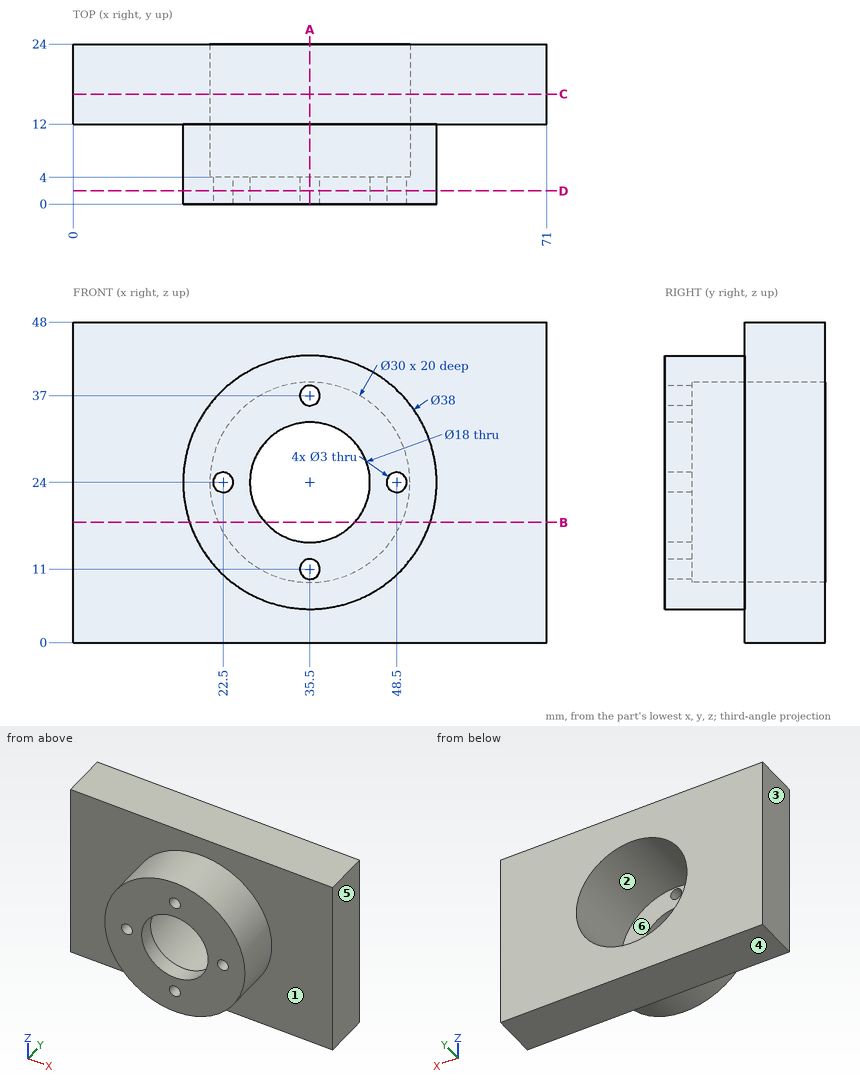
Input: dimensioned drawing with shaded views. Units: mm. Origin: part minimum x, y, z. A direction names the side the tool comes from. Give positions to 0.01 mm unless a question says otherwise; leave off trailing zeros. Write each loop counter-clockwise with the first axis right and the second up, starting at its lowest first coordinate (ties: lowest second). Pieces come first, ordered by that corner, then holes. Notation, with made-up numbers: (-32, 79) -> (-2, 79) arc R6 cw to (-2, 90) -> close; hole circle Ø8 at (45, 19.5). An arc over 180 degrees is marked (long way). Return JSON: item names as keys, results as strings. Group by question number.
1. Section B-B, the plane z = 18. Output: boundary loops of the cut face in (x, y), then the cut area to 3 significant figures.
2. Material intervals for line 1 (Z direction, x = 35.5, y = 1.15); line 2 (Z direction, x = 35.5, y = 16); line 3 (Y direction, x = 11, z = 20), sorted ascending. Write a range as from..to.
3. Section D-D, the plane y = 2. Output: boundary loops of the cut face in (x, z).
4. Section C-C, the plane y = 16.5. Output: boundary loops of the cut face in (x, z).
5. Mould query, pull axis X, two halves, no side actions, for the marked faces 4, 5 and 6. Classes: +X half, -X half, draft (parallel to the pull), parting line (faces both ways), or undercut.
6. Access query for the marked faces 1, 2 and 3. Directions: +Z, -Z, +X, -X, +Y, -Y. A direction counts if a zero-diameter tool reaches every point of the face in a straight line with its end or side. Return the directions, or none.
7. Pin query (flat end, axial travel): pin 1 Ø3.5 at (x, z) = (35.5, 11) entering from +Y; pin 2 Ø3 at (x, y) = (31, 5.5) entering from +Z; pin 3 Ø5 at (x, y) = (39.5, 5) entering from +Z. Return the tip coordinate at first contact, or that it passes through.
8. Section A-A, the plane x = 35.5. Output: boundary loops of the cut face in (y, z), then the cut area to 3 significant figures.
Determined:
{
 "1": {"outline": "(0, 12) -> (17.47, 12) -> (17.47, 0) -> (28.79, 0) -> (28.79, 4) -> (21.75, 4) -> (21.75, 24) -> (0, 24) -> close; (42.21, 0) -> (53.53, 0) -> (53.53, 12) -> (71, 12) -> (71, 24) -> (49.25, 24) -> (49.25, 4) -> (42.21, 4) -> close", "area": "681 mm2"},
 "2": {"line 1": "z = 5..9.5, 12.5..15, 33..35.5, 38.5..43", "line 2": "z = 0..9, 39..48", "line 3": "y = 12..24"},
 "3": {"outline": "circle Ø38 at (35.5, 24); hole circle Ø3 at (22.5, 24); hole circle Ø18 at (35.5, 24); hole circle Ø3 at (35.5, 11); hole circle Ø3 at (35.5, 37); hole circle Ø3 at (48.5, 24)"},
 "4": {"outline": "(0, 0) -> (71, 0) -> (71, 48) -> (0, 48) -> close; hole circle Ø30 at (35.5, 24)"},
 "5": {"face 4": "draft", "face 5": "+X half", "face 6": "undercut"},
 "6": {"face 1": "-Y", "face 2": "+Y", "face 3": "+Z, -Z, -X, +Y, -Y"},
 "7": {"pin 1": "stops at y = 4", "pin 2": "stops at z = 42.76", "pin 3": "stops at z = 42.94"},
 "8": {"outline": "(0, 5) -> (12, 5) -> (12, 0) -> (24, 0) -> (24, 9) -> (4, 9) -> (4, 9.5) -> (0, 9.5) -> close; (0, 12.5) -> (4, 12.5) -> (4, 15) -> (0, 15) -> close; (0, 33) -> (4, 33) -> (4, 35.5) -> (0, 35.5) -> close; (0, 38.5) -> (4, 38.5) -> (4, 39) -> (24, 39) -> (24, 48) -> (12, 48) -> (12, 43) -> (0, 43) -> close", "area": "336 mm2"}
}
